Check sheet for the modelled part. Datum: model origin and axes. Units: mm. A direction names the side the tool comes from. Round coordinates to 2 decimals unless told otherwise and drop trailing zeros. Write each loop counter-clockwise with the first axis right and the second up, starting at its lowest first coordinate (ties: lowest second). Pieces come first, ordered by that corner, then holes. Notation, with made-up numbers: M -27.75,13 L 9.25,13 A14 ccw 9.25,25 Z; hole C 69,39 d2. An arc over 180 degrees is marked long. Answer in a Markdown table with one row per item.
```python
from build123d import *

# Parameters (mm, degrees)
PAD_DEPTH       = 20
SKETCH004_R     = 2
POCKET002_DEPTH = 163.001
SKETCH005_R     = 2
POCKET003_DEPTH = 85.001


with BuildPart() as part:
    # Sketch → Pad (new body)
    with BuildSketch(Plane.XY):
        Polygon((-10, -42.5), (153, -42.5), (153, -30.5), (0, -30.5), (0, 30.5), (153, 30.5), (153, 42.5), (-10, 42.5), (-10, 38.5), (-17, 38.5), (-17, 33.5), (-10, 33.5), (-10, -33.5), (-17, -33.5), (-17, -38.5), (-10, -38.5), align=None)
    extrude(amount=PAD_DEPTH)

    # Sketch004 → Pocket002 (cut, through all)
    with BuildSketch(Plane(origin=(-10, 0, 0), x_dir=(0, -1, 0), z_dir=(-1, 0, 0))):
        with Locations((0, 10)):
            Circle(SKETCH004_R)
    extrude(amount=-POCKET002_DEPTH, mode=Mode.SUBTRACT)

    # Sketch005 → Pocket003 (cut, through all)
    with BuildSketch(Plane.XZ.offset(42.5)):
        with Locations((-5, 10)):
            Circle(SKETCH005_R)
        with Locations((143, 10)):
            Circle(SKETCH005_R)
    extrude(amount=-POCKET003_DEPTH, mode=Mode.SUBTRACT)


solid = part.part
```
1. Section check B-B, the plane y = -19. Record the cut outline in (x, z).
Found:
| item | result |
|---|---|
| outline | M -10,0 L 0,0 L 0,20 L -10,20 Z; hole C -5,10 d4 |
2. Draft check along Y on faces 1 (the face through (153, 36, 10)), 2 (the face through (0, -0.4, 7.6)), 3 (the face through (-13, 38.5, 10)). Enter one of: +Y half, -Y half, draft (parallel to the pull), parting line (faces both ways), or undercut.
Found:
| item | result |
|---|---|
| face 1 | draft |
| face 2 | undercut |
| face 3 | +Y half |
3. Section check A-A, the plane x = 143. Record the cut outline in (y, z), and give its area (3 significant figures).
Found:
| item | result |
|---|---|
| outline | M -42.5,0 L -30.5,0 L -30.5,8 L -42.5,8 Z; M -42.5,12 L -30.5,12 L -30.5,20 L -42.5,20 Z; M 30.5,0 L 42.5,0 L 42.5,8 L 30.5,8 Z; M 30.5,12 L 42.5,12 L 42.5,20 L 30.5,20 Z |
| area | 384 mm2 |
4. Go/stop test with flat-tipped pins: pin 1 (5.5 mm diameter, centred on x = -15, z = 9, fed in from +Y); pin 2 (8 mm diameter, centred on y = -18.5, z = 10, fed in from +X); pin 3 (1.2 mm diameter, centred on y = 41, z = 8, fed in from -X). Record where each tip stops, or that it passes through.
Found:
| item | result |
|---|---|
| pin 1 | stops at y = 38.5 |
| pin 2 | stops at x = 0 |
| pin 3 | stops at x = -10 |
5. Section check C-C, the plane x = 76.5. Record the cut outline in (y, z).
Found:
| item | result |
|---|---|
| outline | M -42.5,0 L -30.5,0 L -30.5,20 L -42.5,20 Z; M 30.5,0 L 42.5,0 L 42.5,20 L 30.5,20 Z |
6. Section check D-D, the plane z = 15.75. Record the cut outline in (x, y), and give its area (3 significant figures).
Found:
| item | result |
|---|---|
| outline | M -17,-38.5 L -10,-38.5 L -10,-42.5 L 153,-42.5 L 153,-30.5 L 0,-30.5 L 0,30.5 L 153,30.5 L 153,42.5 L -10,42.5 L -10,38.5 L -17,38.5 L -17,33.5 L -10,33.5 L -10,-33.5 L -17,-33.5 Z |
| area | 4,590 mm2 |
7. Scan lines: L1, parallel to Y at x = 136, z = 9; L2, parallel to Y at x = -7.05, z = 10; L3, parallel to Z at x = -6, y = 0. Record each from-to range of solid material in increasing order.
Found:
| item | result |
|---|---|
| L1 | y = -42.5 to -30.5, 30.5 to 42.5 |
| L2 | y = -42.5 to -2, 2 to 42.5 |
| L3 | z = 0 to 8, 12 to 20 |
8. Access from +Z, -Z, +X, -X, +Y, -Y to the whole of each face (thin tool, end or side, straight path). Record for faces 4 (the face through (-10, -40, 10)), 5 (the face through (61, 32, 0)), 6 (the face through (141, -37, 10)), 7 (the face through (75, 30.5, 10)), 8 (the face through (-14, 33.5, 10)).
Found:
| item | result |
|---|---|
| face 4 | +Z, -Z, -X, -Y |
| face 5 | -Z, +X, -X, +Y, -Y |
| face 6 | +Y, -Y |
| face 7 | +Z, -Z, +X |
| face 8 | +Z, -Z, -X |
